Autodesk Inventor part; units mm, degrees
ref_plane "YZ Plane" through (0, 0, 0) normal (1, 0, 0) x (0, 1, 0)
ref_plane "XZ Plane" through (0, 0, 0) normal (0, 1, 0) x (-1, 0, 0)
ref_plane "XY Plane" through (0, 0, 0) normal (0, 0, 1) x (1, 0, 0)
ref_plane "Work Plane1" through (0, 0, 0) normal (0, 0, 1) x (1, 0, 0)
sketch "Sketch1" plane through (0, 0, 0) normal (0, 0, 1) x (1, 0, 0)
  line L0 (-75.8806, 15.6994) -> (-120.8806, 15.6994)
  line L1 (-120.8806, 15.6994) -> (-120.8806, -18.8006)
  line L2 (-120.8806, -18.8006) -> (-75.8806, -18.8006)
  line L3 (-75.8806, -18.8006) -> (-75.8806, 15.6994)
  point P0 (0, 0)
  dimension "d0" = 34.5
  dimension "d1" = 45
extrude "Extrusion1" add sketch "Sketch1" along normal blind 8.5
sketch "Sketch2" plane through (0, 0, 8.5) normal (0, 0, 1) x (1, 0, 0)
  line L0 (-120.8806, 15.6994) -> (-120.8806, -18.8006)
  line L1 (-120.8806, -1.5506) -> (-113.8806, -1.5506)
  line L2 (-113.8806, -1.5506) -> (-82.8806, -1.5506)
  line L3 (-82.8806, -1.5506) -> (-82.8806, -4.0506)
  line L4 (-82.8806, -1.5506) -> (-82.8806, 0.9494)
  line L5 (-82.8806, -4.0506) -> (-113.8806, -4.0506)
  line L6 (-113.8806, -4.0506) -> (-113.8806, 0)
  line L7 (-113.8806, 0) -> (-82.8806, 0)
  line L8 (-82.8806, 0) -> (-82.8806, -4.0506)
  line L9 (-82.8806, -4.0506) -> (-113.8806, -4.0506)
  line L10 (-113.8806, -4.0506) -> (-113.8806, 0)
  line L11 (-113.8806, 0) -> (-82.8806, 0)
  line L12 (-82.8806, 0) -> (-82.8806, -4.0506)
  point P0 (0, 0)
  dimension "d4" = 7
  dimension "d5" = 31
  dimension "d6" = 2.5
  dimension "d7" = 2.5
extrude "Extrusion2" cut sketch "Sketch2" against normal blind 2
sketch "Sketch3" plane through (0, 0, 8.5) normal (0, 0, 1) x (1, 0, 0)
  line L0 (-82.8806, 0) -> (-82.8806, -4.0506)
  line L1 (-113.8806, 0) -> (-82.8806, 0)
  line L2 (-113.8806, -4.0506) -> (-113.8806, 0)
  line L3 (-82.8806, -4.0506) -> (-113.8806, -4.0506)
  line L4 (-75.8806, -18.8006) -> (-75.8806, 15.6994)
  line L5 (-82.8806, -2.0253) -> (-79.3754, -2.0253)
  line L6 (-113.8806, -2.0253) -> (-117.3858, -2.0253)
  circle A0 centre (-117.3858, -2.0253) radius 2.0253
  circle A1 centre (-79.3754, -2.0253) radius 2.0253
  point P0 (0, 0)
  dimension "d11" = 3.5052
  dimension "d12" = 3.5052
extrude "Extrusion3" cut sketch "Sketch3" against normal blind 2 contours A1 | A0
properties part number "Breadboard"
Geometry check sheet. Reference: the model listing, model coordinates, mm. A direction names the side the tool comes from. Round coordinates to 2 decimals unless told otherwise and drop trailing zeros. Loops run counter-clockwise (first coordinate to the right, second up) from the corner with the lowest first, then second, coordinate; pieces in that order, holes last.
Item 1: Gauge pin test, flat end, axial feed: pin 1 (3 mm diameter, centred on x = -117.39, y = -2.03, fed in from +Z). Record the tip position at first contact, or that the pin passes through.
Item 2: Thickness scan on line 1 (Y direction, x = -94, z = 7); line 2 (Z direction, x = -116, y = -3). Record the ranges inside material, lowest first.
Item 3: Access from +Z, -Z, +X, -X, +Y, -Y to the whole of each face (thin tool, end or side, straight path). Record for faces 4 (the flat face through (-120.881, -1, 4)), 5 (the flat face through (-98, -4.051, 8)).
Item 4: Cross-section at B-B on x = -108.5. Record the boundary of the cut face in (y, z).
Item 5: Cross-section at A-A on z = 7.5. Record the boundary of the cut face in (x, y), then the cut area to 3 significant figures.
Item 6: Mould release check, pull along Y, two halves, no side actions. Record for faces 1 (the flat face through (-98, 15.699, 4)), 2 (the flat face through (-75.881, -2, 4)), 3 (the cylindrical face through (-80.87, -0.66, 7.51)): pulls with the +Y half, pulls with the -Y half, needs draft (parallel to the pull), parting line crosses it, or undercut.
Item 7: Cross-section at C-C on x = -117. Record the boundary of the cut face in (y, z), then the cut area to 3 significant figures.
Answer sheet:
1. pin 1: stops at z = 6.5
2. line 1: y = -18.8 to -4.05, 0 to 15.7
2. line 2: z = 0 to 6.5
3. face 4: +Z, -Z, -X, +Y, -Y
3. face 5: +Z
4. outline: (-18.8, 0) - (15.7, 0) - (15.7, 8.5) - (0, 8.5) - (0, 6.5) - (-4.05, 6.5) - (-4.05, 8.5) - (-18.8, 8.5) - close
5. outline: (-120.88, -18.8) - (-75.88, -18.8) - (-75.88, 15.7) - (-120.88, 15.7) - close; hole circle Ø4.05 at (-117.39, -2.03); hole (-113.88, -4.05) - (-82.88, -4.05) - (-82.88, 0) - (-113.88, 0) - close; hole circle Ø4.05 at (-79.38, -2.03)
5. area: 1,400 mm2
6. face 1: pulls with the +Y half
6. face 2: needs draft
6. face 3: undercut
7. outline: (-18.8, 0) - (15.7, 0) - (15.7, 8.5) - (-0.04, 8.5) - (-0.04, 6.5) - (-4.01, 6.5) - (-4.01, 8.5) - (-18.8, 8.5) - close
7. area: 285 mm2
